```python
from build123d import *

# Parameters (mm, degrees)
IZIM1_W                     = 400
IZIM1_H                     = 200
IZIM1_R                     = 2
Y_KSEKLIK_EKSTR_ZYON1_DEPTH = 1.75
IZIM2_W                     = 390
IZIM2_H                     = 180.5
Y_KSEKLIK_EKSTR_ZYON2_DEPTH = 24.953
IZIM4_W                     = 378
IZIM4_H                     = 182.48
Y_KSEKLIK_EKSTR_ZYON4_DEPTH = 68.7


with BuildPart() as part:
    # Çizim1 → Yükseklik-Ekstrüzyon1 (new, symmetric)
    with BuildSketch(Plane.XY):
        Rectangle(IZIM1_W, IZIM1_H)
        with Locations((-195, 95)):
            Circle(IZIM1_R, mode=Mode.SUBTRACT)
        with Locations((-65, 95)):
            Circle(IZIM1_R, mode=Mode.SUBTRACT)
        with Locations((65, 95)):
            Circle(IZIM1_R, mode=Mode.SUBTRACT)
        with Locations((195, 95)):
            Circle(IZIM1_R, mode=Mode.SUBTRACT)
        with Locations((-65, -95)):
            Circle(IZIM1_R, mode=Mode.SUBTRACT)
        with Locations((65, -95)):
            Circle(IZIM1_R, mode=Mode.SUBTRACT)
        with Locations((195, -95)):
            Circle(IZIM1_R, mode=Mode.SUBTRACT)
        with Locations((-195, -95)):
            Circle(IZIM1_R, mode=Mode.SUBTRACT)
    extrude(amount=Y_KSEKLIK_EKSTR_ZYON1_DEPTH, both=True)

    # Çizim2 → Yükseklik-Ekstrüzyon2 (add)
    with BuildSketch(Plane.XY.offset(1.75)):
        Rectangle(IZIM2_W, IZIM2_H)
    extrude(amount=Y_KSEKLIK_EKSTR_ZYON2_DEPTH)

    # Çizim4 → Yükseklik-Ekstrüzyon4 (add)
    with BuildSketch(Plane(origin=(0, 0, -1.75), x_dir=(-1, 0, 0), z_dir=(0, 0, -1))):
        Rectangle(IZIM4_W, IZIM4_H)
    extrude(amount=Y_KSEKLIK_EKSTR_ZYON4_DEPTH)


solid = part.part
```
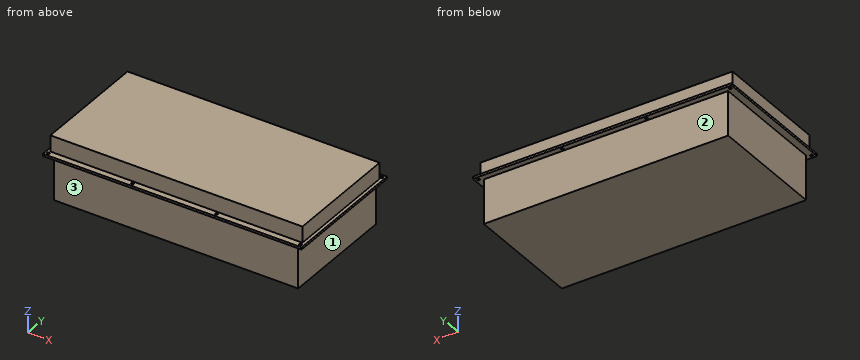
CAD build for the part. Positions are in the model's coordinates, mm. Face numbers are marked on the shaded views. A direction names the side the tool comes from. Round coordinates to 2 decimals unless told otherwise and drop trailing zeros. Loops run counter-clockwise (first coordinate to the right, second up) from the corner with the lowest first, then second, coordinate; pieces in that order, holes last. Notation, with made-up numbers: M 59.5,11.25 L 107.5,11.25 A13 cw 107.5,16.25 Z; hole C 6.25,89 d5. An arc over 180 degrees is marked long. Return JSON: item names as keys, results as strings. Group by question number.
(1) Saw through at A-A, the plane y = -56.5. List the corners of the cut face in (x, z), and give its area (3 significant figures).
(2) Saw through at C-C, the plane z = -31.5. List the corners of the cut face in (x, y).
(3) Drop flat-ended pins along their axis: P1, Ø2, axis at x = 113.5, z = -38, coming from the -Y side; P2, Ø4.5, axis at x = -195, y = 95, coming from the +Z side; P3, Ø20, axis at y = -15, z = 19.5, coming from the +X side. Give the stop position or say it passes through.
(4) Tool access for the marked faces 1, 2 and 3: list every direction of +Z, -Z, +X, -X, +Y, -Y with a clear straight run to the whole face (end or side of a thin tool).
(5) Wall check: probe 1 along Y at (x, z) = (-195, 0); probe 2 along X at (y, z) = (38, -17); probe 3 along Y at (x, z) = (56.5, -41). Give the ranges that are in metal, low to high. Write a range as [from, to].
(6) Saw through at B-B, the plane x = 49. List the corners of the cut face in (y, z), and give its area (3 significant figures).
Answer list:
{
 "1": {"outline": "M -200,-1.75 L -189,-1.75 L -189,-70.45 L 189,-70.45 L 189,-1.75 L 200,-1.75 L 200,1.75 L 195,1.75 L 195,26.7 L -195,26.7 L -195,1.75 L -200,1.75 Z", "area": "37,100 mm2"},
 "2": {"outline": "M -189,-91.24 L 189,-91.24 L 189,91.24 L -189,91.24 Z"},
 "3": {"P1": "y = -91.24", "P2": "z = 1.75", "P3": "x = 195"},
 "4": {"face 1": "-Z, +X, +Y, -Y", "face 2": "-Z, +X, -X, +Y", "face 3": "-Z, +X, -X, -Y"},
 "5": {"probe 1": "[-100, -97], [-93, 93], [97, 100]", "probe 2": "[-189, 189]", "probe 3": "[-91.24, 91.24]"},
 "6": {"outline": "M -100,-1.75 L -91.24,-1.75 L -91.24,-70.45 L 91.24,-70.45 L 91.24,-1.75 L 100,-1.75 L 100,1.75 L 90.25,1.75 L 90.25,26.7 L -90.25,26.7 L -90.25,1.75 L -100,1.75 Z", "area": "17,700 mm2"}
}
